```python
from build123d import *

# Parameters (mm, degrees)
SKETCH1_W           = 215.5
SKETCH1_H           = 201
BOSS_EXTRUDE1_DEPTH = 15
BOSS_EXTRUDE1_DRAFT = -1
FILLET1_R           = 3
CAVITY1_START       = 16.930808083
CAVITY1_DEPTH       = 78.999015724
CAVITY1_START_2     = 92.359823807
CAVITY1_2_DEPTH     = 3.57


with BuildPart() as part:
    # Sketch1 → Boss-Extrude1 (with draft: the straight prism first)
    with BuildSketch(Plane(origin=(0, 0, 0), x_dir=(1, 0, 0), z_dir=(0, 1, 0))):
        Rectangle(SKETCH1_W, SKETCH1_H)
    extrude(amount=BOSS_EXTRUDE1_DEPTH)
    # Boss-Extrude1: the draft: its side faces are tilted about the plane it starts from
    boss_extrude1_sides = [part.faces().sort_by_distance(p)[0] for p in [
        (0, 7.5, 100.5),
        (107.75, 7.5, 0),
        (0, 7.5, -100.5),
        (-107.75, 7.5, 0),
    ]]
    draft(boss_extrude1_sides, Plane(origin=(0, 0, 0), x_dir=(1, 0, 0), z_dir=(0, 1, 0)), BOSS_EXTRUDE1_DRAFT)

    # Fillet1
    fillet1_edges = [part.edges().sort_by_distance(p)[0] for p in [
        (0, 0, 100.5),
        (-107.75, 0, 0),
        (0, 0, -100.5),
        (107.75, 0, 0),
        (107.880912987, 7.5, 100.630912987),
        (-107.880912987, 7.5, 100.630912987),
        (-107.880912987, 7.5, -100.630912987),
        (107.880912987, 7.5, -100.630912987),
    ]]
    fillet(fillet1_edges, radius=FILLET1_R)

    # Cavity1: read off the stored shape, not the designer's step
    # Cavity1 outline → Cavity1 (cut)
    with BuildSketch(Plane.XY.offset(CAVITY1_START)):
        with BuildLine():
            ThreePointArc((-10.617650831, 15), (-2.951958482, 11.347239001), (4.713733868, 15))
            Line((4.713733868, 15), (-10.617650831, 15))
        make_face()
    extrude(amount=CAVITY1_DEPTH, mode=Mode.SUBTRACT)

    # Cavity1 2 outline → Cavity1 2 (cut)
    with BuildSketch(Plane.XY.offset(CAVITY1_START_2)):
        with BuildLine():
            Line((8.860541518, 15), (4.713733868, 15))
            ThreePointArc((4.713733868, 15), (-2.951958482, 11.347239001), (-10.617650831, 15))
            Line((-10.617650831, 15), (-14.764458482, 15))
            Line((-14.764458482, 15), (-14.764458482, 12.397239001))
            Line((-14.764458482, 12.397239001), (-9.251958482, 6.044739001))
            ThreePointArc((-9.251958482, 6.044739001), (-2.951958482, 3.104739001), (3.348041518, 6.044739001))
            Line((3.348041518, 6.044739001), (8.860541518, 12.397239001))
            Line((8.860541518, 12.397239001), (8.860541518, 15))
        make_face()
    extrude(amount=CAVITY1_2_DEPTH, mode=Mode.SUBTRACT)

    # Cavity1 3 outline → Cavity1 3 (revolve, cut)
    with BuildSketch(Plane(origin=(-2.951958482, 21.217239001, 0), x_dir=(1, 0, 0), z_dir=(0, -1, 0))):
        with BuildLine():
            ThreePointArc((6.217239001, 11.929675453), (8.859575731, 13.83427815), (9.87, 16.930808083))
            Line((9.87, 16.930808083), (6.217239001, 16.930808083))
            Line((6.217239001, 16.930808083), (6.217239001, 11.929675453))
        make_face()
    revolve(axis=Axis((-2.951958482, 21.217239001, 0), (0, 0, 1)), mode=Mode.SUBTRACT)


solid = part.part
```
Verification items for the finished model (mm, model axes). A direction names the side the tool comes from. Give positions to 0.01 mm unless a question says otherwise; leave off trailing zeros.
1. Set-up check for faces 3 (the flat face through (-1, 0, -1)), 4 (the flat face through (-3, 10, 95.93)): record each of +Z, -Z, +X, -X, +Y, -Y from which the full face is reachable in a straight line by a thin tool's end or side.
2. Go/stop test with flat-tipped pins: pin 1 Ø6 at (x, y) = (-4.5, 10.5) entering from +Z; pin 2 Ø3.5 at (x, y) = (-1, 8) entering from -Z; pin 3 Ø0.8 at (y, z) = (13, 94.5) entering from -X. Record where each tip stops, or that it passes through.
3. Thickness scan on line 1 (X direction, y = 12.75, z = -8.5); line 2 (X direction, y = 3.5, z = -75); line 3 (Z direction, x = 1, y = 6.75). Record the ranges inside material, lowest first.
4. Mould release check, pull along X, two halves, no side actions. Record for faces 1 (the flat face through (-2, 15, -1)), 2 (the cylindrical face through (-3.075, 11.348, 54.117)): released by +X, released by -X, zero draft, split by the parting line, or undercut.
Geometry says:
1. face 3: +Z, -Z, +X, -X, -Y
1. face 4: +Y
2. pin 1: stops at z = 100.74
2. pin 2: stops at z = -100.67
2. pin 3: stops at x = -107.98
3. line 1: x = -107.97 to 107.97
3. line 2: x = -107.81 to 107.81
3. line 3: z = -100.62 to 92.36, 95.93 to 100.62
4. face 1: zero draft
4. face 2: undercut
